Here's the drawing with two shaded views (mm, measured from the low corner). I have some questions. Give positions to 0.01 mm unless a question says otherwise; leave off trailing zeros. Loops run counter-clockwise (first coordinate to the right, second up) from the corner with the lowest first, then second, coordinate; pieces in that order, holes last. Notation, with made-up numbers: (51.5, 75.5) -> (76.5, 75.5) arc R6 cw to (76.5, 82.5) -> close; hole circle Ø2 at (68, 35.5). An arc over 180 degrees is marked (long way). Write each question's results on one line, items separated by ' | '. Start each with the question number.
Q1. Will these pins go through, and if not, where does the flat tip stop? P1, Ø1.7, axis at x = 3, z = 28.5, coming from the +Y side; P2, Ø0.5, axis at x = 2.5, y = 3.5, coming from the +Z side.
Q2. If I drill on line 1 along Z through (x, y) = (2.65, 3.2); line 2 along Y through (x, z) = (2.1, 32.5); line 3 along Y through (x, z) = (0.55, 2), over which ranges is the centre line in solid material (lowest first)?
Q3. If we section it at A-A, the plane x = 2: List the corners of the cut face in (y, z) for me, plus the area to 3 significant figures.
Q4. If we section it at D-D, the plane z = 28: List the corners of the cut face in (x, y) for me.
Q5. If we section it at C-C, the plane z = 16.5: List the corners of the cut face in (x, y) for me.
Q6. If we section it at B-B, the plane y = 0.8: List the corners of the cut face in (x, z) for me.
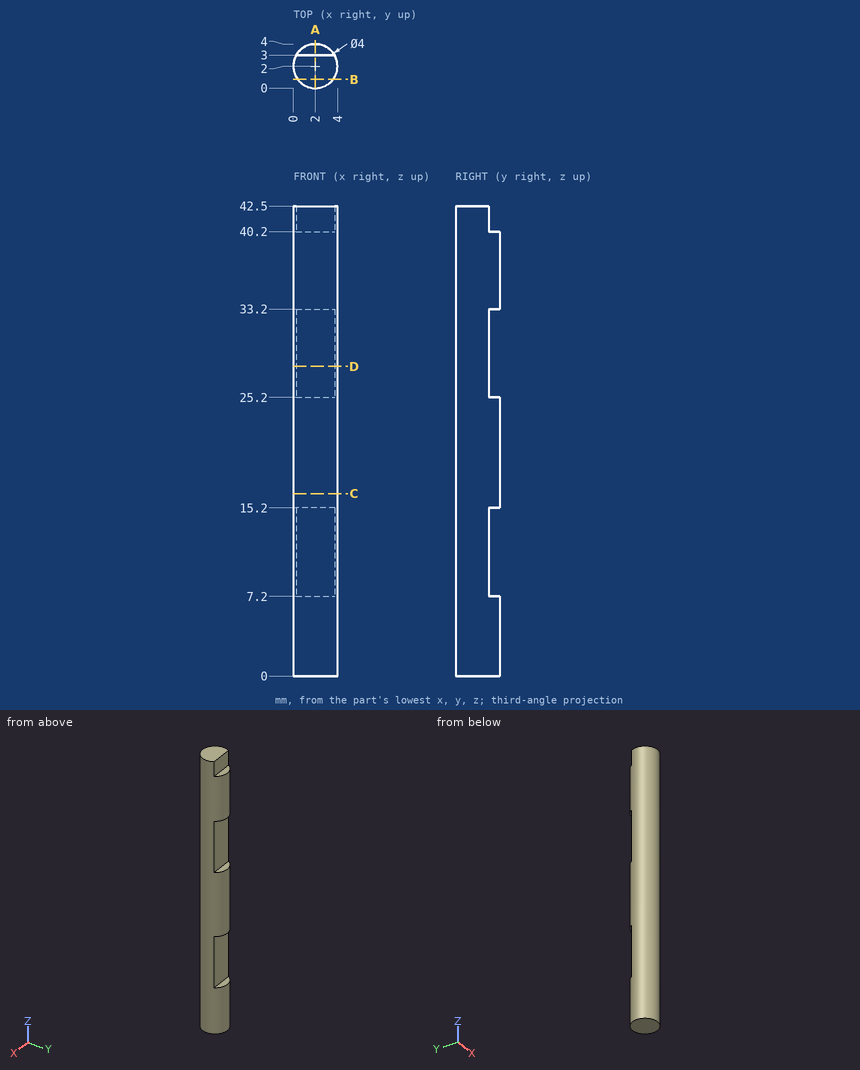
Final values:
1) P1: stops at y = 3 | P2: stops at z = 40.2
2) line 1: z = 0 to 7.2, 15.2 to 25.2, 33.2 to 40.2 | line 2: y = 0 to 3 | line 3: y = 0.62 to 3.38
3) outline: (0, 0) -> (4, 0) -> (4, 7.2) -> (3, 7.2) -> (3, 15.2) -> (4, 15.2) -> (4, 25.2) -> (3, 25.2) -> (3, 33.2) -> (4, 33.2) -> (4, 40.2) -> (3, 40.2) -> (3, 42.5) -> (0, 42.5) -> close | area: 152 mm²
4) outline: (0.27, 3) arc R2 ccw (long way) to (3.73, 3) -> close
5) outline: circle Ø4 at (2, 2)
6) outline: (0.4, 0) -> (3.6, 0) -> (3.6, 42.5) -> (0.4, 42.5) -> close
